```python
from build123d import *

# Parameters (mm, degrees)
BOSS_EXTRUDE4_DEPTH            = 40
CUT_EXTRUDE1_REACH             = 42
SKETCH6_R                      = 30
CUT_EXTRUDE1_DIRECTION_2_DEPTH = 1.0000001


with BuildPart() as part:
    # Sketch2 → Boss-Extrude4 (new body)
    with BuildSketch(Plane(origin=(0, 0, 0), x_dir=(1, 0, 0), z_dir=(0, 1, 0))):
        with BuildLine():
            Line((200, 30), (-250, 30))
            Line((-250, 30), (-250, -30))
            Line((-250, -30), (250, -30))
            Line((250, -30), (250, 30))
            Line((250, 30), (250, 112.573687244))
            add(Edge.make_bspline(
                [(250, 112.573687244), (257.32553359, 114.720346637), (264.651067179, 116.867006031)],
                knots=[0, 0, 0, 0.441237609, 0.441237609, 0.441237609], degree=2))
            ThreePointArc((264.651067179, 116.867006031), (316.316425408, 174.744880654), (243.415537745, 148.200235436))
            add(Edge.make_bspline(
                [(200, 130), (221.707768873, 139.100117718), (243.415537745, 148.200235436)],
                knots=[0, 0, 0, 0.816012756, 0.816012756, 0.816012756], degree=2))
            Line((200, 130), (200, 30))
        make_face()
    extrude(amount=BOSS_EXTRUDE4_DEPTH)

    # Sketch6 → Cut-Extrude1 (cut, up to next)
    with BuildSketch(Plane.XZ, mode=Mode.PRIVATE) as cut_extrude1_sk1:
        with Locations((283.204484122, -152.303861418)):
            Circle(SKETCH6_R)
    cut_extrude1_tool1 = extrude(cut_extrude1_sk1.sketch, amount=-CUT_EXTRUDE1_REACH, mode=Mode.PRIVATE) & part.part
    add(cut_extrude1_tool1.solids().sort_by_distance((283.204484, 0, -152.303861))[0], mode=Mode.SUBTRACT)

    # Sketch6 → Cut-Extrude1 direction 2 (cut)
    with BuildSketch(Plane.XZ):
        with Locations((283.204484122, -152.303861418)):
            Circle(SKETCH6_R)
    extrude(amount=CUT_EXTRUDE1_DIRECTION_2_DEPTH, mode=Mode.SUBTRACT)


solid = part.part
```
The listing builds one solid part. Answer for the finished solid, in the listing's coordinates (mm). A direction names the side the tool comes from. Coordinates: 2 decimals unless noted, no trailing zeros. Write each loop counter-clockwise with the first axis right and the second up, starting at its lowest first coordinate (ties: lowest second). Pieces come first, ordered by that corner, then holes. Notation, with made-up numbers: (20, 1.5) - (72, 1.5) arc R16 cw to (72, 7.5) - close; hole circle Ø2 at (55.5, 56). An arc over 180 degrees is marked (long way). Return JSON: item names as keys, results as strings. Group by question number.
Q1. For a pull along Z with two mould halves and no side action, classify faces 1 (the cylindrical face through (311.82, 19.72, -143.29)), 2 (the flat face through (-22, 20, -30)), 3 (the flat face through (56, 40, -24)), 4 (the flat face through (-3, 20, 30)) as +Z half, -Z half, draft (parallel to the pull), parting line (faces both ways), or undercut.
Q2. Find the intervals of material crossed by line 1 along X through (y, z) = (37, -151.5); line 2 along Z through (x, y) = (190, 18); line 3 along Z through (x, y) = (266.5, 3.5), in increasing order. Write a range as [from, to].
Q3. The part is cut by section A-A on x = 284. Write down the section's boundary in (y, z).
Q4. Which of the six approach directions +Z, -Z, +X, -X, +Y, -Y give full straight-line access (tool end or side, diameter ignored) to faces 5 (the flat face through (200, 20, -81)), 6 (the flat face through (56, 0, -24))?
Q5. Flat-ended cylindrical pins translate along their axes: pin 1 Ø20 at (x, y) = (2, 14.5) entering from -Z; pin 2 Ø12 at (y, z) = (8.5, -39) entering from -X; pin 3 Ø1.5 at (y, z) = (24.5, -67) entering from +X. Find the tip coordinate at first contact, or state that the pin passes through.
Q6. The part is cut by section B-B on x = -51. Write down the section's boundary in (y, z), and give its area (3 significant figures).
Q7. The part is cut by section C-C on z = -90. Write down the section's boundary in (x, y), and give its area (3 significant figures).
Evaluation:
{
 "1": {"face 1": "undercut", "face 2": "-Z half", "face 3": "draft", "face 4": "+Z half"},
 "2": {"line 1": "x = [243.21, 253.22], [313.19, 323.2]", "line 2": "z = [-30, 30]", "line 3": "z = [-188.65, -177.22], [-127.38, -115.96]"},
 "3": {"outline": "(0, -192.3) - (40, -192.3) - (40, -182.29) - (0, -182.29) - close; (0, -122.31) - (40, -122.31) - (40, -112.31) - (0, -112.31) - close"},
 "4": {"face 5": "-Z, -X, +Y, -Y", "face 6": "+Z, -Z, +X, -X, -Y"},
 "5": {"pin 1": "stops at z = -30", "pin 2": "stops at x = 200", "pin 3": "stops at x = 250"},
 "6": {"outline": "(0, -30) - (40, -30) - (40, 30) - (0, 30) - close", "area": "2,400 mm2"},
 "7": {"outline": "(200, 0) - (250, 0) - (250, 40) - (200, 40) - close", "area": "2,000 mm2"}
}
